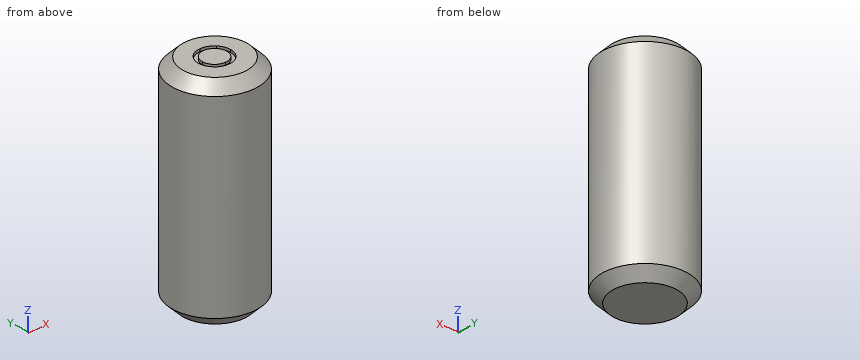
```python
from build123d import *

# Parameters (mm, degrees)
SKETCH1_R           = 4
BOSS_EXTRUDE1_DEPTH = 10
CHAMFER1_SIZE       = 1
CUT_EXTRUDE2_DEPTH  = 0.25


with BuildPart() as part:
    # Sketch1 → Boss-Extrude1 (new, symmetric)
    with BuildSketch(Plane(origin=(0, 0, 0), x_dir=(0, 1, 0), z_dir=(0, 0, 1))):
        with Locations(Location((0, 0, 0), (0, 0, 270))):
            Circle(SKETCH1_R)
    extrude(amount=BOSS_EXTRUDE1_DEPTH, both=True)

    # Chamfer1
    chamfer1_edges = [part.edges().sort_by_distance(p)[0] for p in [
        (-4, 0, -10),
        (-4, 0, 10),
    ]]
    chamfer(chamfer1_edges, length=CHAMFER1_SIZE)

    # Sketch4 → Cut-Extrude2 (cut)
    with BuildSketch(Plane.XY.offset(10)):
        with BuildLine():
            add(Edge.make_bspline(
                [(0.00617457, 1.571131981), (0.061021739, 1.569964106), (0.168563633, 1.567674187), (0.32605836, 1.543199941), (0.476395658, 1.505774381), (0.620151307, 1.454035453), (0.755484216, 1.384684653), (0.884365637, 1.301931177), (1.006442219, 1.203893927), (1.079611395, 1.128056135), (1.116751493, 1.089561468)],
                knots=[0, 0, 0, 0, 1.054011418, 2.066658804, 3.057071809, 4.030435133, 4.997543892, 5.974964718, 6.972108034, 8, 8, 8, 8], degree=3))
            add(Edge.make_bspline(
                [(1.116751493, 1.089561468), (1.148730869, 1.052745485), (1.212070732, 0.979826008), (1.293288697, 0.861591022), (1.363256194, 0.739145192), (1.419328149, 0.610862533), (1.463539605, 0.477862909), (1.494928972, 0.339689182), (1.513599755, 0.1966465), (1.516117432, 0.099499256), (1.517392519, 0.050298648)],
                knots=[0, 0, 0, 0, 1.025258237, 2.030674902, 3.01204498, 3.988269485, 4.97094183, 5.956517959, 6.965070386, 8, 8, 8, 8], degree=3))
            add(Edge.make_bspline(
                [(1.517392519, 0.050298648), (1.51627099, 0.000812868), (1.514054798, -0.096973342), (1.493090665, -0.240995474), (1.46048371, -0.3806467), (1.413818752, -0.51534235), (1.353980913, -0.645494153), (1.280962984, -0.770533638), (1.194252564, -0.890707504), (1.095962282, -1.004995319), (0.987331567, -1.110328136), (0.86948454, -1.202131873), (0.744737073, -1.280785044), (0.611430384, -1.344140947), (0.470781827, -1.39409489), (0.322488035, -1.429180623), (0.166779383, -1.450393976), (0.060462559, -1.45311806), (0.00617457, -1.454509044)],
                knots=[0, 0, 0, 0, 0.998656419, 1.973391657, 2.932242238, 3.890759089, 4.846373663, 5.82037756, 6.809684879, 7.83454468, 8.860553229, 9.859544525, 10.845671541, 11.83227036, 12.833544569, 13.85385346, 14.904124723, 16, 16, 16, 16], degree=3))
            add(Edge.make_bspline(
                [(0.00617457, -1.454509044), (-0.048379395, -1.453113392), (-0.155226092, -1.450379935), (-0.311484357, -1.42926304), (-0.460043921, -1.39411106), (-0.600876605, -1.343976783), (-0.734756431, -1.280783019), (-0.860226713, -1.202369659), (-0.978169473, -1.11030091), (-1.08682317, -1.005002697), (-1.18510729, -0.890705604), (-1.2718193, -0.770534131), (-1.344836815, -0.645494024), (-1.404674763, -0.515342384), (-1.451339692, -0.380646691), (-1.483946655, -0.240995477), (-1.504910786, -0.096973341), (-1.507126978, 0.000812868), (-1.508248507, 0.050298648)],
                knots=[0, 0, 0, 0, 1.099876186, 2.154163076, 3.173186993, 4.173200201, 5.163417411, 6.152872554, 7.150605724, 8.17532212, 9.198891216, 10.186952605, 11.159729845, 12.11414092, 13.071450619, 14.029093627, 15.002601286, 16, 16, 16, 16], degree=3))
            add(Edge.make_bspline(
                [(-1.508248507, 0.050298648), (-1.506964724, 0.099231843), (-1.504423053, 0.19611116), (-1.485771043, 0.338884944), (-1.454504121, 0.476824817), (-1.410239668, 0.609311075), (-1.353650879, 0.737031574), (-1.28466655, 0.859779952), (-1.202620112, 0.977480295), (-1.139532168, 1.05030553), (-1.107607481, 1.087157622)],
                knots=[0, 0, 0, 0, 1.031353054, 2.041901799, 3.029428768, 4.008703097, 4.981709435, 5.96992636, 6.972712378, 8, 8, 8, 8], degree=3))
            add(Edge.make_bspline(
                [(-1.107607481, 1.087157622), (-1.070523377, 1.125986124), (-0.997590961, 1.202349206), (-0.874906701, 1.300100662), (-0.746342334, 1.384576175), (-0.609513847, 1.452548992), (-0.465876295, 1.506078727), (-0.314768589, 1.543296459), (-0.156739429, 1.567586007), (-0.04867129, 1.56993821), (0.00617457, 1.571131981)],
                knots=[0, 0, 0, 0, 1.027980169, 2.021703884, 2.998553061, 3.971491411, 4.943284454, 5.930300938, 6.949603206, 8, 8, 8, 8], degree=3))
        make_face()
        with BuildLine():
            add(Edge.make_bspline(
                [(0.004572006, 1.212157622), (-0.034213836, 1.211055232), (-0.110784268, 1.208878909), (-0.223492365, 1.192325875), (-0.331995398, 1.166100156), (-0.43649922, 1.128838377), (-0.536651417, 1.08072535), (-0.632547877, 1.021630081), (-0.724470665, 0.952335274), (-0.810621595, 0.872949363), (-0.889687095, 0.786230513), (-0.958804782, 0.693832388), (-1.017576332, 0.597253707), (-1.066536514, 0.496394037), (-1.103001872, 0.390231278), (-1.129485326, 0.2799677), (-1.146022744, 0.165378652), (-1.148178605, 0.087480345), (-1.149274148, 0.047894802)],
                knots=[0, 0, 0, 0, 1.021534396, 2.016698045, 2.994645724, 3.958388632, 4.93408049, 5.916473867, 6.921342795, 7.962252576, 8.998418191, 10.008913653, 10.997312074, 11.973003931, 12.956656626, 13.948281152, 14.957379055, 16, 16, 16, 16], degree=3))
            add(Edge.make_bspline(
                [(-1.149274148, 0.047894802), (-1.147437778, -0.003250372), (-1.143792927, -0.104763978), (-1.114152657, -0.254262404), (-1.064568337, -0.397784521), (-0.997611446, -0.534488962), (-0.913718625, -0.660971566), (-0.814876263, -0.773738976), (-0.702145177, -0.871094189), (-0.576869176, -0.951872299), (-0.441607099, -1.016054877), (-0.298457018, -1.06153942), (-0.149153367, -1.091107069), (-0.047118246, -1.094045897), (0.004572006, -1.095534685)],
                knots=[0, 0, 0, 0, 1.016792936, 2.018143844, 3.017858371, 4.030088057, 5.03801393, 6.028138512, 7.003788237, 7.991172063, 8.984598303, 9.972568034, 10.972917682, 12, 12, 12, 12], degree=3))
            add(Edge.make_bspline(
                [(0.004572006, -1.095534685), (0.056259285, -1.094037222), (0.158288537, -1.091081272), (0.307384739, -1.061688335), (0.450143564, -1.01585558), (0.58526515, -0.951944483), (0.710484125, -0.870787437), (0.824025978, -0.77428872), (0.922024391, -0.66067289), (1.005834225, -0.534321429), (1.073887646, -0.397996455), (1.123239876, -0.254235915), (1.152951403, -0.104770724), (1.156586636, -0.003252632), (1.15841816, 0.047894802)],
                knots=[0, 0, 0, 0, 1.02726834, 2.027799167, 3.010890988, 4.004497153, 4.992059811, 5.971914811, 6.958719428, 7.966827853, 8.981595046, 9.981490638, 10.983022906, 12, 12, 12, 12], degree=3))
            add(Edge.make_bspline(
                [(1.15841816, 0.047894802), (1.157322994, 0.087480582), (1.155167875, 0.165379354), (1.138625059, 0.279965015), (1.112161585, 0.390241126), (1.075622594, 0.496357701), (1.026875149, 0.597514849), (0.966970243, 0.693548823), (0.898134785, 0.78655059), (0.818115218, 0.872669036), (0.732054215, 0.952366221), (0.640094172, 1.021656952), (0.54433991, 1.080465632), (0.444478673, 1.129249907), (0.339961453, 1.165761153), (0.231610448, 1.192477303), (0.119383237, 1.208808957), (0.043087187, 1.211034261), (0.004572006, 1.212157622)],
                knots=[0, 0, 0, 0, 1.042956736, 2.052379634, 3.044323526, 4.02829302, 5.004299113, 5.996692471, 7.007513377, 8.048758398, 9.090003419, 10.095195979, 11.07790575, 12.047570684, 13.018257071, 13.989683339, 14.985167495, 16, 16, 16, 16], degree=3))
        make_face(mode=Mode.SUBTRACT)
    extrude(amount=-CUT_EXTRUDE2_DEPTH, mode=Mode.SUBTRACT)


solid = part.part
```
CAD build for the part. Positions are in the model's coordinates, mm. Give positions to 0.01 mm unless a question says otherwise; leave off trailing zeros. Write each loop counter-clockwise with the first axis right and the second up, starting at its lowest first coordinate (ties: lowest second). Pieces come first, ordered by that corner, then holes. Notation, with made-up numbers: M 69,53 L 92,53 A15 cw 92,63 Z; hole C 33.25,43.5 d11. An arc over 180 degrees is marked long. Return JSON: item names as keys, results as strings. Group by question number.
(1) Drill centre lines: L1, parallel to Y at x = -3, z = 3.5; L2, parallel to X at y = -2.25, z = 0; L3, parallel to X at y = -3.5, z = -5.5. Where is each one in solid material? Low to high. Write a range as [from, to].
(2) Band-saw the part on A-A (z = -8.5). Give the cut face in (x, y), and give its area (3 significant figures).
(3) Flat gauge pins, fed straight in: pin 1 Ø3 at (x, z) = (2.5, -7.5) entering from -Y; pin 2 Ø3 at (y, z) = (-0.5, -8) entering from -X; pin 3 Ø2 at (y, z) = (2, -5) entering from +X. Where does each tip first touch, or does it go through?
Entries:
{
 "1": {"L1": "y = [-2.65, 2.65]", "L2": "x = [-3.31, 3.31]", "L3": "x = [-1.94, 1.94]"},
 "2": {"outline": "C 0,0 d8", "area": "50.3 mm^2"},
 "3": {"pin 1": "stops at y = -3.87", "pin 2": "stops at x = -4", "pin 3": "stops at x = 3.87"}
}
